```python
from build123d import *

# Parameters (mm, degrees)
SKETCH_R     = 80
SKETCH_R_2   = 53
SKETCH_R_3   = 2.25
PAD_DEPTH    = 4
SKETCH001_R  = 2.762237
POCKET_DEPTH = 4.001
FILLET_R     = 2


with BuildPart() as part:
    # Sketch → Pad (new body)
    with BuildSketch(Plane.XY):
        Circle(SKETCH_R)
        Circle(SKETCH_R_2, mode=Mode.SUBTRACT)
        with Locations((25, 63)):
            Circle(SKETCH_R_3, mode=Mode.SUBTRACT)
        with Locations((-47.25, 46.5)):
            Circle(SKETCH_R_3, mode=Mode.SUBTRACT)
        with Locations((-41.25, -55)):
            Circle(SKETCH_R_3, mode=Mode.SUBTRACT)
        with Locations((41.25, -55)):
            Circle(SKETCH_R_3, mode=Mode.SUBTRACT)
    extrude(amount=PAD_DEPTH)

    # Sketch001 (on Face8 of Pad) → Pocket (cut, through all)
    with BuildSketch(Plane.XY.offset(4)):
        with Locations((0, -53.138237)):
            Circle(SKETCH001_R)
    extrude(amount=-POCKET_DEPTH, mode=Mode.SUBTRACT)

    # Fillet
    fillet_edges = [part.edges().sort_by_distance(p)[0] for p in [
        (-80, 0, 4),
    ]]
    fillet(fillet_edges, radius=FILLET_R)


solid = part.part
```
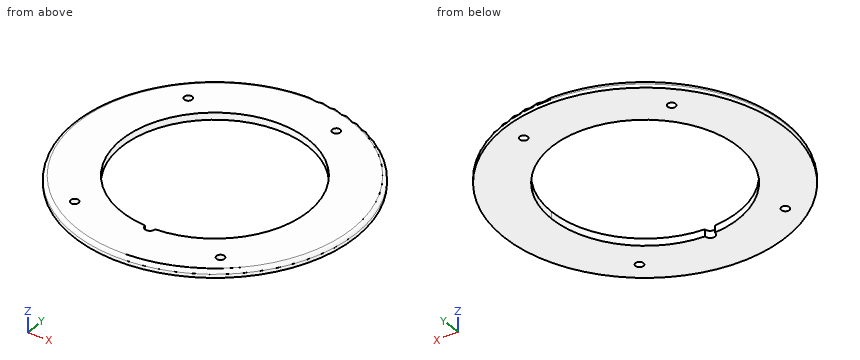
CAD build for the part. Positions are in the model's coordinates, mm. Round coordinates to 2 decimals unless told otherwise and drop trailing zeros. One line per question, with ' | ' between items.
1. Probe L1, parallel to Y at x = -41.25, z = 1.3; L2, parallel to Y at x = 41.25, z = 2.55; L3, parallel to X at y = -7.5, z = 0.65. List the from-to ranges inside material, lowest first. Write a range as from..to.
Working result:
L1: -68.55..-57.25, -52.75..-33.28, 33.28..68.55 | L2: -68.46..-57.25, -52.75..-33.28, 33.28..68.46 | L3: -79.65..-52.47, 52.47..79.65
2. Cut at A-A on x = -41.25. Count the separate pieces of the cut face and the enclosed holes in it, and give its area (3 significant figures).
Working result:
separate pieces: 3 | enclosed holes: 0 | area: 262 mm2
3. Pin check, flat tips, straight feed: pin 1 Ø2.5 at (x, y) = (41.25, -55) entering from -Z; pin 2 Ø1 at (y, z) = (-61, 3) entering from +X. Stop position of each tip, or through.
Working result:
pin 1: through | pin 2: x = 52.04
